```python
from build123d import *

# Parameters (mm, degrees)
BOSS_EXTRUDE1_DEPTH = 20
SKETCH2_R           = 5
CUT_EXTRUDE1_DEPTH  = 21
SKETCH3_R           = 15
BOSS_EXTRUDE2_DEPTH = 20
CHAMFER1_SIZE       = 2


with BuildPart() as part:
    # Sketch1 → Boss-Extrude1 (new body)
    with BuildSketch(Plane(origin=(0, 0, 0), x_dir=(1, 0, 0), z_dir=(0, 1, 0))):
        with BuildLine():
            Line((-100, 45), (100, 45))
            ThreePointArc((100, 45), (145, 0), (100, -45))
            Line((100, -45), (-100, -45))
            ThreePointArc((-100, -45), (-145, 0), (-100, 45))
        make_face()
    extrude(amount=BOSS_EXTRUDE1_DEPTH)

    # Sketch2 → Cut-Extrude1 (cut, through all)
    with BuildSketch(Plane(origin=(0, 20, 0), x_dir=(1, 0, 0), z_dir=(0, 1, 0))):
        with Locations((-135, 0)):
            Circle(SKETCH2_R)
        with Locations((-100, 35)):
            Circle(SKETCH2_R)
        with Locations((-65, 0)):
            Circle(SKETCH2_R)
        with Locations((-100, -35)):
            Circle(SKETCH2_R)
        with Locations((-75.251262658, 24.748737342)):
            Circle(SKETCH2_R)
    extrude(amount=-CUT_EXTRUDE1_DEPTH, mode=Mode.SUBTRACT)

    # Sketch3 → Boss-Extrude2 (add)
    with BuildSketch(Plane.XZ):
        with Locations((100, 0)):
            Circle(SKETCH3_R)
    extrude(amount=BOSS_EXTRUDE2_DEPTH)

    # Chamfer1
    chamfer1_edges = [part.edges().sort_by_distance(p)[0] for p in [
        (145, 20, 0),
        (0, 20, -45),
        (-145, 20, 0),
        (0, 0, -45),
        (145, 0, 0),
        (0, 0, 45),
        (-145, 0, 0),
        (0, 20, 45),
    ]]
    chamfer(chamfer1_edges, length=CHAMFER1_SIZE)


solid = part.part
```
The listing builds one solid part. Answer for the finished solid, in the listing's coordinates (mm). A direction names the side the tool comes from. Round coordinates to 2 decimals unless told otherwise and drop trailing zeros. Loops run counter-clockwise (first coordinate to the right, second up) from the corner with the lowest first, then second, coordinate; pieces in that order, holes last. Notation, with made-up numbers: (-38.5, -23.5) - (5.5, -23.5) arc R14 ccw to (5.5, -14.5) - close; hole circle Ø1 at (-9.75, -1.75). An arc over 180 degrees is marked (long way). Return JSON: item names as keys, results as strings. Group by question number.
1. Which of the six approach directions +Z, -Z, +X, -X, +Y, -Y give full straight-line access (tool end or side, diameter ignored) to faces 1 (the cylindrical face through (114.307, -9.86, 4.506)), 2 (the cylindrical face through (-80.246, 10.14, -24.969))?
2. The part is cut by section C-C on y = -13. Determine the outline of the cut face in (x, z).
3. Consider probe 1 along X at (y, z) = (9.5, 0); probe 2 along Z at (x, y) = (-100, 4); probe 3 along Z at (x, y) = (-65, 8.5). Determine where each line is inside the solid, lowest interval first.
4. Each of these flat-tipped pins is pushed along its axis until it touches: P1, Ø13, axis at x = -135, z = 0, coming from the -Y side; P2, Ø9, axis at x = -100, z = -35, coming from the +Y side; P3, Ø12, axis at y = -11.5, z = 10.5, coming from the +X side; P4, Ø5, axis at y = 1.5, z = 22.5, coming from the +X side. Where does it stop, or does it pass through?
5. The part is cut by section A-A on x = -65. Determine the outline of the cut face in (y, z).
6. The part is cut by section B-B on y = 11.5. Determine the outline of the cut face in (x, z).
7. The mould has two halves that part along Z. Classify faces 3 (the flat face through (100, -20, 0)), 4 (the conical face through (-143.31, 0.32, 0.95)), 5 (the cylindrical face through (-95.381, 10.14, 36.915)): pulls with the +Z half, pulls with the -Z half, needs draft (parallel to the pull), parting line crosses it, or undercut.
Resolved:
{
 "1": {"face 1": "-Y", "face 2": "+Y, -Y"},
 "2": {"outline": "circle Ø30 at (100, 0)"},
 "3": {"probe 1": "x = -145 to -140, -130 to -70, -60 to 145", "probe 2": "z = -45 to -40, -30 to 30, 40 to 45", "probe 3": "z = -45 to -5, 5 to 45"},
 "4": {"P1": "stops at y = 0", "P2": "passes through", "P3": "stops at x = 114.31", "P4": "stops at x = 140.29"},
 "5": {"outline": "(0, -43) - (2, -45) - (18, -45) - (20, -43) - (20, -5) - (0, -5) - close; (0, 5) - (20, 5) - (20, 43) - (18, 45) - (2, 45) - (0, 43) - close"},
 "6": {"outline": "(-100, -45) - (100, -45) arc R45 ccw to (100, 45) - (-100, 45) arc R45 ccw to start; hole circle Ø10 at (-135, 0); hole circle Ø10 at (-100, -35); hole circle Ø10 at (-100, 35); hole circle Ø10 at (-75.25, -24.75); hole circle Ø10 at (-65, 0)"},
 "7": {"face 3": "needs draft", "face 4": "parting line crosses it", "face 5": "undercut"}
}
